Source: CAD feature listing. Evaluate the final solid. Frame: model axes, mm. Face numbers are marked on the shaded views. A direction names the side the tool comes from. Give positions to 0.01 mm unless a question says otherwise; leave off trailing zeros. Order: outer loops, then holes, each group sorted by start corner. A loop starts at its lowest first (then second) coordinate and runs counter-clockwise, first axis right, second up. Notation, with made-up numbers: (81.5, 58.25) -> (116.5, 58.25) arc R15 ccw to (116.5, 66.25) -> close; hole circle Ø8 at (49.5, 36.25). An arc over 180 degrees is marked (long way). Use one line per item in the form item = value. Start each with the question number.
from build123d import *

# Parameters (mm, degrees)
F0_R     = 2.3
F0_R_2   = 1.15
F1_DEPTH = 8
F0_R_3   = 18.5
F0_R_4   = 16.5
F2_DEPTH = 8
F3_DEPTH = 1.8
F4_R     = 2
F6_DEPTH = 1.801


with BuildPart() as f1:
    # F0 (on Front) → F1 (new body)
    with BuildSketch(Plane.XZ):
        Circle(F0_R)
        Circle(F0_R_2, mode=Mode.SUBTRACT)
    extrude(amount=F1_DEPTH)



with BuildPart() as f2:
    # F0 (on Front) → F2 (new body)
    with BuildSketch(Plane.XZ):
        with Locations((0, 0.311320764)):
            Circle(F0_R_3)
        Circle(F0_R_4, mode=Mode.SUBTRACT)
    extrude(amount=F2_DEPTH)


with BuildPart() as f1_1:
    add(f1.part)

    add(f2.part)  # F3 merges F2
    # F0 (on Front) → F3 (join)
    with BuildSketch(Plane.XZ):
        with Locations((0, 0.311320764)):
            Circle(F0_R_3)
        Circle(F0_R_4, mode=Mode.SUBTRACT)
        Circle(F0_R_4)
        Circle(F0_R, mode=Mode.SUBTRACT)
        Circle(F0_R)
        Circle(F0_R_2, mode=Mode.SUBTRACT)
        Circle(F0_R_2)
    extrude(amount=F3_DEPTH)

    # F4
    f4_edges = [f1_1.edges().sort_by_distance(p)[0] for p in [
        (-16.5, -1.8, 0),
        (-2.3, -1.8, 0),
    ]]
    fillet(f4_edges, radius=F4_R)

    # F5 (on face) → F6 (cut, through all)
    with BuildSketch(Plane.XZ.offset(1.8)):
        with BuildLine():
            Line((1.4706866163, 4.0406782694), (4.9592920782, 13.6255430014))
            ThreePointArc((4.9592920782, 13.6255430014), (0, 14.5), (-4.9592920782, 13.6255430014))
            Line((-4.9592920782, 13.6255430014), (-1.4706866163, 4.0406782694))
            ThreePointArc((-1.4706866163, 4.0406782694), (0, 4.3), (1.4706866163, 4.0406782694))
        make_face()
        with BuildLine():
            ThreePointArc((14.4911669918, -0.5060427022), (14.4977915798, -0.2530598933), (14.5, 0))
            ThreePointArc((14.5, 0), (13.7100193462, 4.7207382396), (11.4261559273, 8.9270913922))
            Line((11.4261559273, 8.9270913922), (3.3884462405, 2.6473443439))
            ThreePointArc((3.3884462405, 2.6473443439), (4.0657298751, 1.3999430642), (4.3, 0))
            ThreePointArc((4.3, 0), (4.2993450892, -0.0750453477), (4.2973805562, -0.1500678358))
            Line((4.2973805562, -0.1500678358), (14.4911669918, -0.5060427022))
        make_face()
        with BuildLine():
            ThreePointArc((3.9967416593, -13.9382945911), (8.5228861582, -11.7307464184), (12.021044802, -8.1082971003))
            Line((12.021044802, -8.1082971003), (3.564861562, -2.4045294849))
            ThreePointArc((3.564861562, -2.4045294849), (2.5274765849, -3.4787730758), (1.18524063, -4.1334252925))
            Line((1.18524063, -4.1334252925), (3.9967416593, -13.9382945911))
        make_face()
        with BuildLine():
            ThreePointArc((-12.021044802, -8.1082971003), (-8.5228861582, -11.7307464184), (-3.9967416593, -13.9382945911))
            Line((-3.9967416593, -13.9382945911), (-1.18524063, -4.1334252925))
            ThreePointArc((-1.18524063, -4.1334252925), (-2.5274765849, -3.4787730758), (-3.564861562, -2.4045294849))
            Line((-3.564861562, -2.4045294849), (-12.021044802, -8.1082971003))
        make_face()
        with BuildLine():
            Line((-3.3884462405, 2.6473443439), (-11.4261559273, 8.9270913922))
            ThreePointArc((-11.4261559273, 8.9270913922), (-13.7903194863, 4.4807464184), (-14.4911669918, -0.5060427022))
            Line((-14.4911669918, -0.5060427022), (-4.2973805562, -0.1500678358))
            ThreePointArc((-4.2973805562, -0.1500678358), (-4.0895430201, 1.3287730758), (-3.3884462405, 2.6473443439))
        make_face()
    extrude(amount=-F6_DEPTH, mode=Mode.SUBTRACT)


solid = f1_1.part
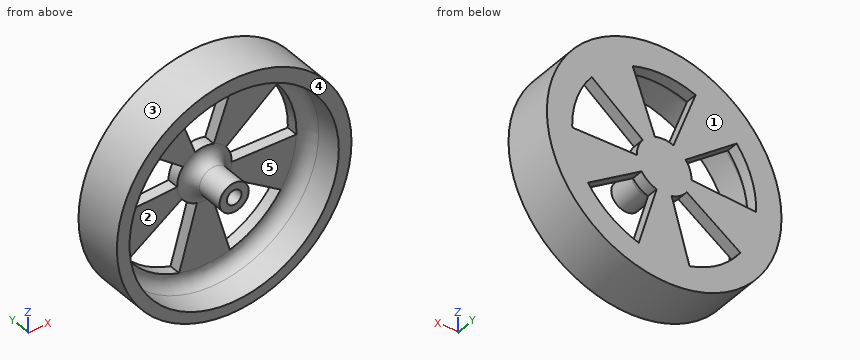
1) Material intervals for probe 1 along Z at (x, y) = (0, -4); probe 2 along X at (y, z) = (-6.8, 0); probe 3 along Z at (x, y) = (-10, -0.5), sorted ascending.
2) Cut plane A-A, the plane x = 0. Return the cut outline in (y, z).
3) Cut plane B-B, the plane y = -6. Return the cut outline in (x, z), plus the area to 3 significant figures.
4) Cut plane C-C, the plane z = 6.5. Count the separate pieces of the cut face and the enclosed holes in it, plus the area to 3 significant figures.
5) Cut plane D-D, the plane y = -0.5. Return the cut outline in (x, z).
6) Draft query along X for the marked faces 1, 2 and 3. Return one class per face: +X half, -X half, draft (parallel to the pull), parting line (faces both ways), or undercut.
7) Reachability of the marked faces 4 and 5 from +Z, -Z, +X, -X, +Y, -Y: full face, straight path, thin tool, end or side. Return the list, or none.
8) Pin query (flat end, axial travel): pin 1 (3 mm diameter, centred on y = -6, z = 11, fed in from -X); pin 2 (3 mm diameter, centred on x = -4.5, z = 5.5, fed in from -Y); pin 3 (8 mm diameter, centred on x = -3, z = 4.5, fed in from +Y); pin 4 (1 mm diameter, centred on x = 14, z = 5, fed in from -Y). Return the tip coordinate at first contact, or that it passes through.
Output values:
q1.probe_1 = -18.19 to -16.5, -2.3 to -1.15, 1.15 to 2.3, 16.5 to 18.81
q1.probe_2 = -18.5 to -16.5, -2.3 to -1.15, 1.15 to 2.3, 16.5 to 18.5
q1.probe_3 = -15.25 to -10.5, -6.75 to -0.35, 7.81 to 15.88
q2.outline = (-8, -18.19) -> (0, -18.19) -> (0, 4.3) -> (-1.8, 4.3) arc R2 cw to (-3.8, 2.3) -> (-8, 2.3) -> (-8, 1.15) -> (-1.8, 1.15) -> (-1.8, -1.15) -> (-8, -1.15) -> (-8, -2.3) -> (-3.8, -2.3) arc R2 cw to (-1.8, -4.3) -> (-1.8, -14.5) arc R2 cw to (-3.8, -16.5) -> (-8, -16.5) -> close; (-8, 16.5) -> (-3.8, 16.5) arc R2 cw to (-1.8, 14.5) -> (0, 14.5) -> (0, 18.81) -> (-8, 18.81) -> close
q3.outline = circle Ø37 at (0, 0.31); circle Ø4.6 at (0, 0); hole circle Ø33 at (0, 0); hole circle Ø2.3 at (0, 0)
q3.area = 232 mm^2
q4.separate_pieces = 4
q4.enclosed_holes = 0
q4.area = 67.5 mm^2
q5.outline = circle Ø37 at (0, 0.31); hole (-14.49, -0.51) -> (-4.3, -0.15) arc R4.3 cw to (-3.39, 2.65) -> (-11.43, 8.93) arc R14.5 ccw to start; hole (-12.02, -8.11) arc R14.5 ccw to (-4, -13.94) -> (-1.19, -4.13) arc R4.3 cw to (-3.56, -2.4) -> close; hole (-4.96, 13.63) -> (-1.47, 4.04) arc R4.3 cw to (1.47, 4.04) -> (4.96, 13.63) arc R14.5 ccw to start; hole (1.19, -4.13) -> (4, -13.94) arc R14.5 ccw to (12.02, -8.11) -> (3.56, -2.4) arc R4.3 cw to start; hole (3.39, 2.65) arc R4.3 cw to (4.3, -0.15) -> (14.49, -0.51) arc R14.5 ccw to (11.43, 8.93) -> close
q6.face_1 = draft
q6.face_2 = undercut
q6.face_3 = parting line
q7.face_4 = +Z, -Z, +X, -X, -Y
q7.face_5 = -Y
q8.pin_1 = -16.06
q8.pin_2 = -1.8
q8.pin_3 = 0
q8.pin_4 = -2
